```python
from build123d import *

# Parameters (mm, degrees)
SKETCH2_W               = 40
SKETCH2_H               = 26
SKETCH2_R               = 1.3
SKETCH2_W_2             = 8.6
SKETCH2_H_2             = 8.6
BOSS_EXTRUDE1_DEPTH     = 1.5
SKETCH3_W               = 4
SKETCH3_H               = 26
BOSS_EXTRUDE2_DEPTH     = 1.5
SKETCH5_R               = 1.3
CUT_EXTRUDE1_DEPTH      = 25.04163056
CUT_EXTRUDE3_DEPTH      = 24.900836805
CUT_EXTRUDE3_DEPTH_BACK = 24.900836805
SKETCH6_W               = 1.75
SKETCH6_H               = 2.4
SKETCH7_R               = 1.6
CUT_EXTRUDE4_DEPTH      = 2


with BuildPart() as part:
    # Sketch2 → Boss-Extrude1 (new body)
    with BuildSketch(Plane(origin=(0, 0, 0), x_dir=(1, 0, 0), z_dir=(0, 1, 0))):
        Rectangle(SKETCH2_W, SKETCH2_H)
        with Locations(Location((-10.5, -2.5, 0), (0, 0, 270))):
            Circle(SKETCH2_R, mode=Mode.SUBTRACT)
        with Locations(Location((-10.5, 10, 0), (0, 0, 270))):
            Circle(SKETCH2_R, mode=Mode.SUBTRACT)
        with Locations(Location((10.5, 10, 0), (0, 0, 270))):
            Circle(SKETCH2_R, mode=Mode.SUBTRACT)
        with Locations(Location((10.5, -2.5, 0), (0, 0, 270))):
            Circle(SKETCH2_R, mode=Mode.SUBTRACT)
        with Locations((0, -2.5)):
            Rectangle(SKETCH2_W_2, SKETCH2_H_2, mode=Mode.SUBTRACT)
    extrude(amount=BOSS_EXTRUDE1_DEPTH)

    # Sketch3 → Boss-Extrude2 (add)
    with BuildSketch(Plane(origin=(0, 1.5, 0), x_dir=(1, 0, 0), z_dir=(0, 1, 0))):
        with Locations((-10.5, 0)):
            Rectangle(SKETCH3_W, SKETCH3_H)
        with Locations((10.5, 0)):
            Rectangle(SKETCH3_W, SKETCH3_H)
    extrude(amount=BOSS_EXTRUDE2_DEPTH)

    # Sketch5 → Cut-Extrude1 (cut, through all)
    with BuildSketch(Plane.XZ):
        with Locations(Location((-10.5, 2.5, 0), (0, 0, 90))):
            Circle(SKETCH5_R)
        with Locations(Location((10.5, -10, 0), (0, 0, 270))):
            Circle(SKETCH5_R)
        with Locations(Location((10.5, 2.5, 0), (0, 0, 270))):
            Circle(SKETCH5_R)
        with Locations(Location((-10.5, -10, 0), (0, 0, 90))):
            Circle(SKETCH5_R)
    extrude(amount=-CUT_EXTRUDE1_DEPTH, mode=Mode.SUBTRACT)

    # Sketch6 → Cut-Extrude3 (cut, two sides: drawn at the far end of the back side and taken through both)
    with BuildSketch(Plane(origin=(0, 1.5, 0), x_dir=(1, 0, 0), z_dir=(0, 1, 0)).offset(-CUT_EXTRUDE3_DEPTH_BACK)):
        with Locations((-7.875, 7.5)):
            Rectangle(SKETCH6_W, SKETCH6_H)
    extrude(amount=CUT_EXTRUDE3_DEPTH + CUT_EXTRUDE3_DEPTH_BACK, mode=Mode.SUBTRACT)

    # Sketch7 → Cut-Extrude4 (cut)
    with BuildSketch(Plane(origin=(0, 1.5, 0), x_dir=(1, 0, 0), z_dir=(0, 1, 0))):
        with Locations(Location((16.25, 7.5, 0), (0, 0, 270))):
            Circle(SKETCH7_R)
        with Locations(Location((16.25, -7.5, 0), (0, 0, 270))):
            Circle(SKETCH7_R)
        with Locations(Location((-16.25, -7.5, 0), (0, 0, 270))):
            Circle(SKETCH7_R)
        with Locations(Location((-16.25, 7.5, 0), (0, 0, 270))):
            Circle(SKETCH7_R)
    extrude(amount=-CUT_EXTRUDE4_DEPTH, mode=Mode.SUBTRACT)


solid = part.part
```
Source: CAD feature listing. Evaluate the final solid. Frame: model axes, mm. A direction names the side the tool comes from. Round coordinates to 2 decimals unless told otherwise and drop trailing zeros. Loops run counter-clockwise (first coordinate to the right, second up) from the corner with the lowest first, then second, coordinate; pieces in that order, holes last. Notation, with made-up numbers: M 85.5,50 L 118.5,50 A15 ccw 118.5,66 Z; hole C -4.75,-34 d9. An arc over 180 degrees is marked long. Use a Markdown table: item, result. Add a question column.
1. Cut plane D-D, the plane z = -7.5. Output: boundary loops of the cut face in (x, y).
2. Set-up query: faces 1 (the flat face through (-12.5, 2, 0)), 2 (the flat face through (0, 0, -3)), 3 (the flat face through (16, 1.5, 0)), 4 (the flat face through (-8.5, 2, 3)), 5 (the flat face through (-7, 1, -7)). Return all of +Z, -Z, +X, -X, +Y, -Y with unobstructed straight access to the full face (end or side cutting, diameter ignored); none if empty.
3. Contact query for flat-ended pins moving along their axis: pin 1 (0.8 mm diameter, centred on y = 2.5, z = 0.5, fed in from +X); pin 2 (3.5 mm diameter, centred on x = 16.25, z = -7.5, fed in from +Y); pin 3 (0.8 mm diameter, centred on y = 2, z = -1.5, fed in from -X). Output: stop coordinate, or through.
4. Pull-direction query (Z, two-part tool) for faces 6 (the flat face through (-8, 1, -8.7)), 7 (the flat face through (10, 3, 0)); classes: +Z half, -Z half, draft (parallel to the pull), parting line (faces both ways), or undercut.
5. Cut plane A-A, the plane x = 16.25. Output: boundary loops of the cut face in (y, z), and give its area (3 significant figures).
6. Cut plane C-C, the plane z = 7.5. Output: boundary loops of the cut face in (x, y).
7. Cut plane B-B, the plane y = 2.55. Output: boundary loops of the cut face in (x, z).
8. Ray query, line 1 along X through (y, z) = (0.45, -7.5); line 2 along Z through (x, y) = (-10.5, 1.5); line 3 along X through (y, z) = (2.4, 6). Return the intervals inside material, ascending. Write a range as [from, to].
Solution:
| question | item | result |
|---|---|---|
| 1 | outline | M -20,0 L -17.85,0 L -17.85,1.5 L -20,1.5 Z; M -14.65,0 L -8.75,0 L -8.75,3 L -12.5,3 L -12.5,1.5 L -14.65,1.5 Z; M -7,0 L 14.65,0 L 14.65,1.5 L 12.5,1.5 L 12.5,3 L 8.5,3 L 8.5,1.5 L -7,1.5 Z; M 17.85,0 L 20,0 L 20,1.5 L 17.85,1.5 Z |
| 2 | face 1 | +Z, -Z, -X, +Y |
| 2 | face 2 | +Z, -Z, +X, -X, -Y |
| 2 | face 3 | +Z, -Z, +X, +Y |
| 2 | face 4 | +Z, -Z, +Y |
| 2 | face 5 | +Y, -Y |
| 3 | pin 1 | stops at x = 12.5 |
| 3 | pin 2 | stops at y = 1.5 |
| 3 | pin 3 | stops at x = -12.5 |
| 4 | face 6 | undercut |
| 4 | face 7 | draft |
| 5 | outline | M 0,-13 L 1.5,-13 L 1.5,-9.1 L 0,-9.1 Z; M 0,-5.9 L 1.5,-5.9 L 1.5,5.9 L 0,5.9 Z; M 0,9.1 L 1.5,9.1 L 1.5,13 L 0,13 Z |
| 5 | area | 29.4 mm2 |
| 6 | outline | M -20,0 L -17.85,0 L -17.85,1.5 L -20,1.5 Z; M -14.65,0 L 14.65,0 L 14.65,1.5 L 12.5,1.5 L 12.5,3 L 8.5,3 L 8.5,1.5 L -8.5,1.5 L -8.5,3 L -12.5,3 L -12.5,1.5 L -14.65,1.5 Z; M 17.85,0 L 20,0 L 20,1.5 L 17.85,1.5 Z |
| 7 | outline | M -12.5,-13 L -8.5,-13 L -8.5,-8.7 L -8.75,-8.7 L -8.75,-6.3 L -8.5,-6.3 L -8.5,13 L -12.5,13 Z; M 8.5,-13 L 12.5,-13 L 12.5,13 L 8.5,13 Z; hole C -10.5,-10 d2.6; hole C -10.5,2.5 d2.6; hole C 10.5,-10 d2.6; hole C 10.5,2.5 d2.6 |
| 8 | line 1 | x = [-20, -17.85], [-14.65, -8.75], [-7, 14.65], [17.85, 20] |
| 8 | line 2 | z = [-13, -11.3], [-8.7, 1.2], [3.8, 13] |
| 8 | line 3 | x = [-12.5, -8.5], [8.5, 12.5] |
